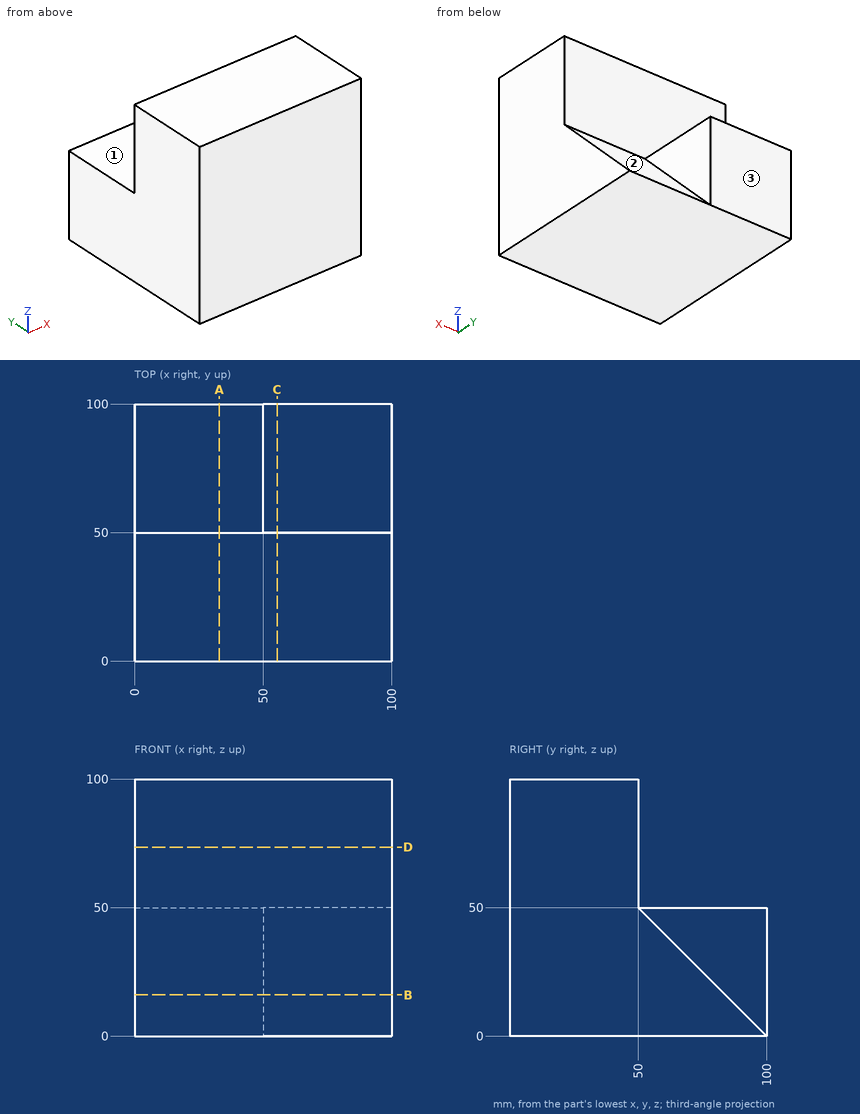
The figure shows three views and two pictorial views of one solid part (mm, origin at its lowest corner). Answer the questions. A direction names the side the tool comes from. Coordinates: 2 decimals unless noted, no trailing zeros. Order: outer loops, then holes, each group sorted by start corner. A loop starts at its lowest first (then second) coordinate and runs counter-clockwise, first axis right, second up.
Q1. A cutting plane is placed at A-A, the plane x = 33. Write down the section's boundary in (y, z), and give its area (3 significant figures).
Q2. Which of the six approach directions +Z, -Z, +X, -X, +Y, -Y give full straight-line access (tool end or side, diameter ignored) to the marked faces 1, 2 and 3?
Q3. Given P1, Ø8, axis at x = 14, z = 25.5, coming from the -Y side; P2, Ø12, axis at x = 13.5, z = 58, coming from the +Y side; P3, Ø8, axis at x = 56.5, z = 16.5, coming from the +Y side; P4, Ø2, axis at x = 43.5, y = 55, coming from the +Z side, each flat-ended and moving along its own axis, determine where each tip first touches the part or whether it passes through.
Q4. Consider line 1 (Y direction, x = 14.5, z = 51); line 2 (Y direction, x = 86.5, z = 36). Determine where each line is inside the solid, lowest interval first.
Q5. A cutting plane is placed at C-C, the plane x = 55.5. Write down the section's boundary in (y, z).
Q6. A cutting plane is placed at B-B, the plane z = 16. Write down the section's boundary in (x, y), and give its area (3 significant figures).
Q7. A cutting plane is placed at D-D, the plane z = 73.5. Write down the section's boundary in (x, y), and give its area (3 significant figures).
Answers follow:
1. outline: (0, 0) - (100, 0) - (100, 50) - (50, 50) - (50, 100) - (0, 100) - close
1. area: 7,500 mm2
2. face 1: +Z, +X, -X, +Y
2. face 2: +Z, +X, +Y
2. face 3: +Z, -Z, +X, -X, +Y
3. P1: stops at y = 0
3. P2: stops at y = 50
3. P3: stops at y = 87.5
3. P4: stops at z = 50
4. line 1: y = 0 to 50
4. line 2: y = 0 to 64
5. outline: (0, 0) - (100, 0) - (50, 50) - (50, 100) - (0, 100) - close
6. outline: (0, 0) - (100, 0) - (100, 84) - (50, 84) - (50, 100) - (0, 100) - close
6. area: 9,200 mm2
7. outline: (0, 0) - (100, 0) - (100, 50) - (0, 50) - close
7. area: 5,000 mm2
